Print and shaded views of the part. All mm, measured from the part's lowest x, y and z. A direction names the side the tool comes from. Coordinates: 2 decimals unless noted, no trailing zeros. Order: outer loops, then holes, each group sorted by start corner. A loop starts at its lowest first (then second) coordinate and runs counter-clockwise, first axis right, second up.
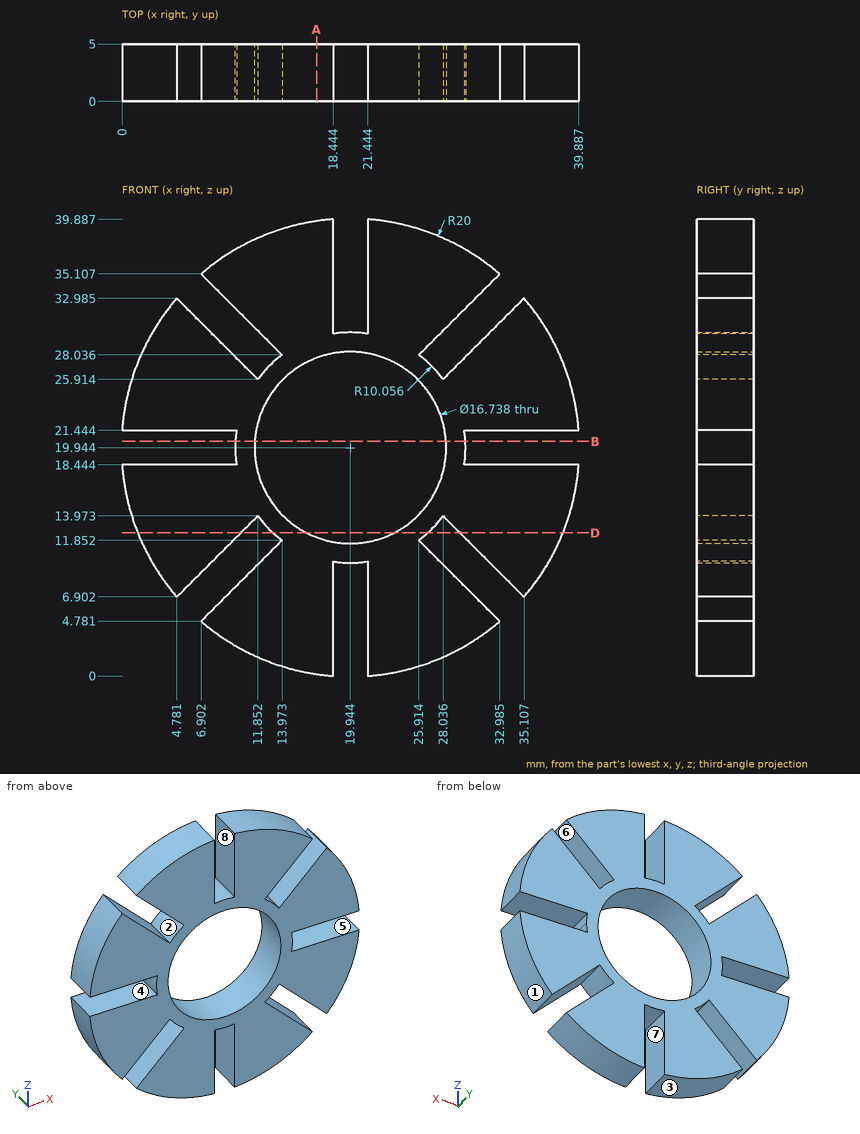
Q1. Mould opens along X. For the marked faces 1, 2 and 3 say: pulls with the +X half, pulls with the -X half, needs draft (parallel to the pull), parting line crosses it, or undercut.
Established:
face 1: pulls with the +X half
face 2: undercut
face 3: pulls with the -X half
Q2. Cut at D-D, the plane z = 12.5. List the corners of the cut face in (x, y) (1 decimal), plus the area to 3 significant figures.
Established:
outline: (1.4, 0) - (10.4, 0) - (10.4, 5) - (1.4, 5) - close; (13.2, 0) - (16.1, 0) - (16.1, 5) - (13.2, 5) - close; (23.8, 0) - (26.7, 0) - (26.7, 5) - (23.8, 5) - close; (29.5, 0) - (38.5, 0) - (38.5, 5) - (29.5, 5) - close
area: 119 mm2
Q3. Drop flat-ended pins along their axis: P1, Ø3, axis at x = 35.5, y = 1.5, coming from the -Z side; P2, Ø2.5, axis at y = 2, z = 36.5, coming from the +X side (1 decimal); P3, Ø2.5, axis at x = 36.5, y = 3.5, coming from the -Z side; P4, Ø10, axis at x = 19.94, z = 19.94, coming from the -Y side. Give the stop position or say it passes through.
Established:
P1: stops at z = 6.9
P2: stops at x = 32.8
P3: stops at z = 7.07
P4: passes through
Q4. Which spindle directions (+Z, -Z, +X, -X, +Y, -Y) get a long thin tool onto all of the face, cutting with end or side? Do the marked faces 4, 5, 6, 7 and 8. Say none if no direction does.
Established:
face 4: -X, +Y, -Y
face 5: +X, +Y, -Y
face 6: +Y, -Y
face 7: -Z, +Y, -Y
face 8: +Z, +Y, -Y
Q5. Cut at A-A, the plane x = 17. List the corners of the cut face in (y, z) (1 decimal).
Established:
outline: (0, 0.2) - (5, 0.2) - (5, 12.1) - (0, 12.1) - close; (0, 27.8) - (5, 27.8) - (5, 39.7) - (0, 39.7) - close
Q6. Cut at B-B, the plane z = 20.5. List the corners of the cut face in (x, y) (1 decimal), plus the area to 3 significant figures.
Established:
outline: (9.9, 0) - (11.6, 0) - (11.6, 5) - (9.9, 5) - close; (28.3, 0) - (30, 0) - (30, 5) - (28.3, 5) - close
area: 16.9 mm2
Q7. Probe line 1 (Z direction, x = 9, y = 4.2) (1 decimal); line 2 (X direction, y = 3.95, z = 13.5) (1 decimal); line 3 (X direction, y = 4.5, z = 20) (1 decimal). List the from-to ranges inside material, lowest first.
Established:
line 1: z = 3.2 to 6.9, 11.1 to 18.4, 21.4 to 28.8, 33 to 36.7
line 2: x = 1 to 11.4, 12.2 to 14.6, 25.3 to 27.7, 28.5 to 38.9
line 3: x = 9.9 to 11.6, 28.3 to 30
